Source: CAD feature listing. Evaluate the final solid. Frame: model axes, mm. Face numbers are marked on the shaded views. A direction names the side the tool comes from. Coordinates: 2 decimals unless noted, no trailing zeros. Write each loop counter-clockwise with the first axis right and the second up, starting at its lowest first coordinate (ties: lowest second). Pieces come first, ordered by that corner, then holes. Notation, with made-up numbers: M -23,1.25 L 35,1.25 A36 cw 35,37.25 Z; hole C -23.75,42.25 d1. An arc over 180 degrees is marked long. One line per item, written item: value. Start each with the question number.
Item 1: Mould query, pull axis X, two halves, no side actions, for the marked faces 3, 4 and 5. Classes: released by +X, released by -X, zero draft, split by the parting line, or undercut.
Item 2: Set-up query: the marked faces 1 and 2. Return all of +Z, -Z, +X, -X, +Y, -Y with unobstructed straight access to the full face (end or side cutting, diameter ignored); none if empty.
Item 3: Cut plane D-D, the plane z = 3.5. Output: boundary loops of the cut face in (x, y).
Item 4: Cut plane C-C, the plane y = 18.5. Output: boundary loops of the cut face in (x, z), then the cut area to 3 significant figures.
Item 5: Cut plane A-A, the plane z = 25. Output: boundary loops of the cut face in (x, y).
Item 6: Cut plane B-B, the plane y = 0. Output: boundary loops of the cut face in (x, z), then the cut area to 3 significant figures.
Item 7: Pin query (flat end, axial travel): P1, Ø20, axis at y = 0, z = 25, coming from the -X side; P2, Ø2, axis at x = -12, z = 27.5, coming from the -Y side; P3, Ø4, axis at x = 3, z = 16, coming from the -Y side; P4, Ø2, axis at x = -8, z = 23, coming from the -Y side. Return the tip coordinate at first contact, or that it passes through.
Item 8: Ray query, L1, parallel to X at y = -10, z = 40; L2, parallel to Z at x = 22.5, y = 0; L3, parallel to Y at x = 21.25, z = 25. Return the intervals inside material, ascending. Write a range as from..to.
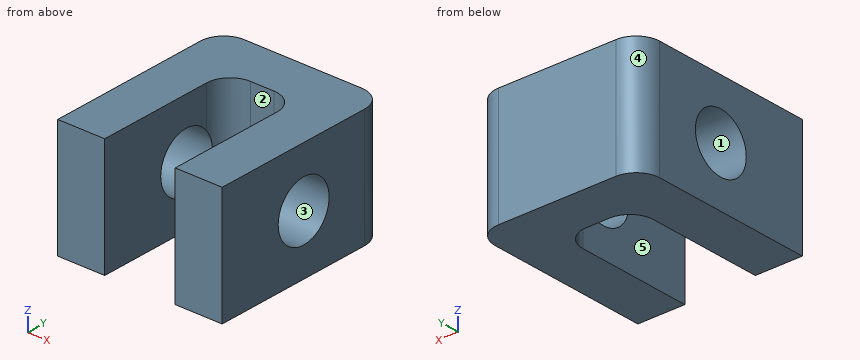
```python
from build123d import *

# Parameters (mm, degrees)
F0_W     = 70
F0_H     = 80
F1_DEPTH = 50
F2_W     = 30
F2_H     = 60
F3_DEPTH = 64
F4_R     = 10
F5_R     = 12.5
F6_DEPTH = 96.7


with BuildPart() as f1:
    # F0 (on Top) → F1 (new body)
    with BuildSketch(Plane.XY):
        Rectangle(F0_W, F0_H)
    extrude(amount=F1_DEPTH)

    # F2 (on face) → F3 (cut)
    with BuildSketch(Plane.XY.offset(50)):
        with Locations((0, -10)):
            Rectangle(F2_W, F2_H)
    extrude(amount=-F3_DEPTH, mode=Mode.SUBTRACT)

    # F4
    f4_edges = [f1.edges().sort_by_distance(p)[0] for p in [
        (35, 40, 25),
        (-35, 40, 25),
        (-15, 20, 25),
        (15, 20, 25),
    ]]
    fillet(f4_edges, radius=F4_R)

    # F5 (on face) → F6 (cut)
    with BuildSketch(Plane(origin=(-35, 0, 0), x_dir=(0, -1, 0), z_dir=(-1, 0, 0))):
        with Locations((0, 25)):
            Circle(F5_R)
    extrude(amount=-F6_DEPTH, mode=Mode.SUBTRACT)


solid = f1.part
```
From the geometry:
1. face 3: zero draft
1. face 4: released by -X
1. face 5: undercut
2. face 1: +X, -X
2. face 2: +Z, -Z, -Y
3. outline: M -35,-40 L -15,-40 L -15,10 A10 cw -5,20 L 5,20 A10 cw 15,10 L 15,-40 L 35,-40 L 35,30 A10 ccw 25,40 L -25,40 A10 ccw -35,30 Z
4. outline: M -35,0 L -10.27,0 L -10.27,50 L -35,50 Z; M 10.27,0 L 35,0 L 35,50 L 10.27,50 Z
4. area: 2,470 mm²
5. outline: M -35,-40 L -15,-40 L -15,-12.5 L -35,-12.5 Z; M -35,12.5 L -14.68,12.5 A10 cw -5,20 L 5,20 A10 cw 14.68,12.5 L 35,12.5 L 35,30 A10 ccw 25,40 L -25,40 A10 ccw -35,30 Z; M 15,-40 L 35,-40 L 35,-12.5 L 15,-12.5 Z
6. outline: M -35,0 L -15,0 L -15,12.5 L -35,12.5 Z; M -35,37.5 L -15,37.5 L -15,50 L -35,50 Z; M 15,0 L 35,0 L 35,12.5 L 15,12.5 Z; M 15,37.5 L 35,37.5 L 35,50 L 15,50 Z
6. area: 1,000 mm²
7. P1: passes through
7. P2: stops at y = 16
7. P3: stops at y = 20
7. P4: stops at y = 19.17
8. L1: x = -35..-15, 15..35
8. L2: z = 0..12.5, 37.5..50
8. L3: y = -40..-12.5, 12.5..40
